Read the model definition and answer for the solid it produces. Units are mm, in the model's axes. A direction names the side the tool comes from. Coordinates: 2 decimals unless noted, no trailing zeros. Order: outer loops, then holes, each group sorted by start corner. A loop starts at its lowest first (then second) coordinate and runs counter-clockwise, first axis right, second up. Notation, with made-up numbers: (16.5, 77.25) - (71.5, 77.25) arc R22 cw to (71.5, 107.25) - close; hole circle Ø1 at (8, 84.5). An arc over 180 degrees is marked (long way). Answer as a JSON object with one key per item and string values. Group by question number.
from build123d import *

# Parameters (mm, degrees)
SKETCH1_W               = 95.25
SKETCH1_H               = 76.2
BOSS_EXTRUDE1_DEPTH     = 9.652
FILLET1_R               = 12.7
CUT_EXTRUDE1_DEPTH      = 62.74877917
CUT_EXTRUDE1_DEPTH_BACK = 62.74877917
SKETCH2_R               = 4.826
SKETCH3_W               = 57.404
SKETCH3_H               = 3.048
CUT_EXTRUDE2_DEPTH      = 91.375559356
SKETCH5_W               = 60.452
SKETCH5_H               = 47.752
BOSS_EXTRUDE2_DEPTH     = 7.874
FILLET2_R               = 7.874
SKETCH6_R               = 3.937
CUT_EXTRUDE3_DEPTH      = 7.874
RIB1_REACH              = 125.976
SKETCH10_WALL_W         = 309.953649084
SKETCH10_WALL_H         = 7.874


with BuildPart() as part:
    # Sketch1 → Boss-Extrude1 (new body)
    with BuildSketch(Plane(origin=(0, 0, 0), x_dir=(1, 0, 0), z_dir=(0, 1, 0))):
        Rectangle(SKETCH1_W, SKETCH1_H)
    extrude(amount=BOSS_EXTRUDE1_DEPTH)

    # Fillet1
    fillet1_edges = [part.edges().sort_by_distance(p)[0] for p in [
        (47.625, 4.826, 38.1),
        (-47.625, 4.826, 38.1),
        (-47.625, 4.826, -38.1),
        (47.625, 4.826, -38.1),
    ]]
    fillet(fillet1_edges, radius=FILLET1_R)

    # Sketch2 → Cut-Extrude1 (cut, two sides: drawn at the far end of the back side and taken through both)
    with BuildSketch(Plane(origin=(0, 9.652, 0), x_dir=(1, 0, 0), z_dir=(0, 1, 0)).offset(-CUT_EXTRUDE1_DEPTH_BACK)):
        with Locations(Location((-34.925, -25.4, 0), (0, 0, 270))):
            Circle(SKETCH2_R)
        with Locations(Location((-34.925, 25.4, 0), (0, 0, 270))):
            Circle(SKETCH2_R)
        with Locations(Location((34.925, 25.4, 0), (0, 0, 270))):
            Circle(SKETCH2_R)
        with Locations(Location((34.925, -25.4, 0), (0, 0, 270))):
            Circle(SKETCH2_R)
    extrude(amount=CUT_EXTRUDE1_DEPTH + CUT_EXTRUDE1_DEPTH_BACK, mode=Mode.SUBTRACT)

    # Sketch3 → Cut-Extrude2 (cut, through all)
    with BuildSketch(Plane.XY.offset(38.1)):
        Rectangle(SKETCH3_W, SKETCH3_H)
    extrude(amount=-CUT_EXTRUDE2_DEPTH, mode=Mode.SUBTRACT)



with BuildPart() as body_2:
    # Sketch5 → Boss-Extrude2 (new body)
    with BuildSketch(Plane(origin=(0, 68.540427062, 39.571834015), x_dir=(0, 0.4999999999999976, -0.86602540378444), z_dir=(0, -0.8660254037844402, -0.4999999999999977))):
        with Locations((32.114183863, 0)):
            Rectangle(SKETCH5_W, SKETCH5_H)
    extrude(amount=-BOSS_EXTRUDE2_DEPTH)

    # Fillet2
    fillet2_edges = [body_2.edges().sort_by_distance(p)[0] for p in [
        (-23.876, 103.120061008, -12.447848887),
        (-23.876, 72.894061008, 39.905118823),
        (23.876, 72.894061008, 39.905118823),
        (23.876, 103.120061008, -12.447848887),
    ]]
    fillet(fillet2_edges, radius=FILLET2_R)

    # Sketch6 → Cut-Extrude3 (cut)
    with BuildSketch(Plane(origin=(0, 75.359511091, 43.508834015), x_dir=(1, 0, 0), z_dir=(0, 0.86602540378444, 0.49999999999999784))):
        with Locations(Location((-16.002, 9.762183863, 0), (0, 0, 270))):
            Circle(SKETCH6_R)
        with Locations(Location((16.002, 9.762183863, 0), (0, 0, 270))):
            Circle(SKETCH6_R)
        with Locations(Location((16.002, 54.466183863, 0), (0, 0, 270))):
            Circle(SKETCH6_R)
        with Locations(Location((-16.002, 54.466183863, 0), (0, 0, 270))):
            Circle(SKETCH6_R)
    extrude(amount=-CUT_EXTRUDE3_DEPTH, mode=Mode.SUBTRACT)


with BuildPart() as part_1:
    add(part.part)

    add(body_2.part)  # Loft1 merges body 2
    # Sketch9 → Loft1 section 0
    with BuildSketch(Plane(origin=(0, 68.540427062, 39.571834015), x_dir=(1, 0, 0), z_dir=(0, -0.86602540378444, -0.49999999999999784))):
        with BuildLine():
            Line((23.876, -49.630618041), (-23.876, -49.630618041))
            Line((-23.876, -49.630618041), (-23.876, -41.756618041))
            Line((-23.876, -41.756618041), (23.876, -41.756618041))
            Line((23.876, -41.756618041), (23.876, -49.630618041))
        make_face()
    # Sketch7 → Loft1 section 1
    with BuildSketch(Plane(origin=(0, 9.652, 0), x_dir=(1, 0, 0), z_dir=(0, 1, 0))):
        with BuildLine():
            Line((-47.625, -3.937), (47.625, -3.937))
            Line((47.625, -3.937), (47.625, 3.937))
            Line((47.625, 3.937), (-47.625, 3.937))
            Line((-47.625, 3.937), (-47.625, -3.937))
        make_face()
    loft()

    # Sketch10 wall → Rib1 (add, up to next)
    with BuildSketch(Plane(origin=(0, 39.483889376, 37.936618823), x_dir=(0, 1, 0), z_dir=(0, 0, 1)), mode=Mode.PRIVATE) as rib1_sk1:
        Rectangle(SKETCH10_WALL_W, SKETCH10_WALL_H)
    rib1_tool1 = extrude(rib1_sk1.sketch, amount=-RIB1_REACH, mode=Mode.PRIVATE) - part_1.part
    add(rib1_tool1.solids().sort_by_distance((0, 39.483889376, 37.936618823))[0])


solid = part_1.part
1. For faces 5 (the cylindrical face through (21.508, 74.064, 37.988)), 6 (the cylindrical face through (-12.1, 77.14, 32.67)), 7 (the flat face through (0, 39, 37.937)), 8 (the flat face through (0, 5, 38.1)), 9 (the cylindrical face through (-21.508, 74.064, 37.988)), determine the directions among +Z, -Z, +X, -X, +Y, -Y from which every point of the face is accessible in a straight line to the end or side of a thin tool.
2. A cutting plane is placed at C-C on z = 5.5. Write down the section's boundary in (x, y) (3 decimals).
3. A cutting plane is placed at A-A on z = -19. Write down the section's boundary in (x, y) (3 decimals), and give its area (3 significant figures).
4. Given pin 1 (6 mm diameter, centred on x = 15.5, y = 87.5, fed in from +Z); pin 2 (5 mm diameter, centred on x = -19, z = 21, fed in from +Y); pin 3 (6 mm diameter, centred on x = -6, z = -20.5, fed in from -Y), each flat-ended and moving along its own axis, determine where each tip first touches the part or whether it passes through.
5. A cutting plane is placed at B-B on z = 23.5. Write down the section's boundary in (x, y) (1 decimal).
6. Straight lines are drawn through the part: L1, parallel to X at y = 5, z = 25 (3 decimals); L2, parallel to X at y = 6.5, z = -25.4 (3 decimals); L3, parallel to X at y = 58, z = 32.5. For each, find the intervals that lie inside material, in ascending order.
7. For a pull along Y with two mould halves and no side action, classify faces 1 (the cylindrical face through (16.18, 78.85, 29.71)), 2 (the cylindrical face through (38.187, 4.758, 21.843)), 3 (the flat face through (0, 1.524, 1)), 4 (the flat face through (10, 9.652, 21)) as pulls with the +Y half, pulls with the -Y half, needs draft (parallel to the pull), parting line crosses it, or undercut.
Derived:
{
 "1": {"face 5": "+Z, +X", "face 6": "none", "face 7": "+Z, +X, -X", "face 8": "+Z, +X, -X, -Y", "face 9": "+Z, -X"},
 "2": {"outline": "(-47.625, 0) - (-28.702, 0) - (-28.702, 1.524) - (28.702, 1.524) - (28.702, 0) - (47.625, 0) - (47.625, 9.652) - (3.937, 9.652) - (3.937, 88.212) - (23.876, 88.212) - (23.876, 97.304) - (-23.876, 97.304) - (-23.876, 88.212) - (-3.937, 88.212) - (-3.937, 9.652) - (-47.625, 9.652) - close"},
 "3": {"outline": "(-47.625, 0) - (-28.702, 0) - (-28.702, 1.524) - (28.702, 1.524) - (28.702, 0) - (47.625, 0) - (47.625, 9.652) - (-47.625, 9.652) - close", "area": "832 mm2"},
 "4": {"pin 1": "stops at z = 27.68", "pin 2": "stops at y = 89.8", "pin 3": "stops at y = 1.52"},
 "5": {"outline": "(-47.6, 0) - (-39.4, 0) - (-39.4, 9.7) - (-47.6, 9.7) - close; (-30.5, 0) - (-28.7, 0) - (-28.7, 1.5) - (28.7, 1.5) - (28.7, 0) - (30.5, 0) - (30.5, 9.7) - (3.9, 9.7) - (3.9, 77.8) - (23.9, 77.8) - (23.9, 86.9) - (-23.9, 86.9) - (-23.9, 77.8) - (-3.9, 77.8) - (-3.9, 9.7) - (-30.5, 9.7) - close; (39.4, 0) - (47.6, 0) - (47.6, 9.7) - (39.4, 9.7) - close"},
 "6": {"L1": "x = -47.625 to -39.734, -30.116 to 30.116, 39.734 to 47.625", "L2": "x = -47.625 to -39.751, -30.099 to 30.099, 39.751 to 47.625", "L3": "x = -3.94 to 3.94"},
 "7": {"face 1": "undercut", "face 2": "needs draft", "face 3": "pulls with the -Y half", "face 4": "undercut"}
}
